Here's the drawing with two shaded views (mm, measured from the low corner). I have some questions. Give positions to 0.01 mm unless a question says otherwise; leave off trailing zeros. Write each loop counter-clockwise with the first axis right and the second up, starting at its lowest first coordinate (ties: lowest second). Pieces come first, ordered by that corner, then holes.
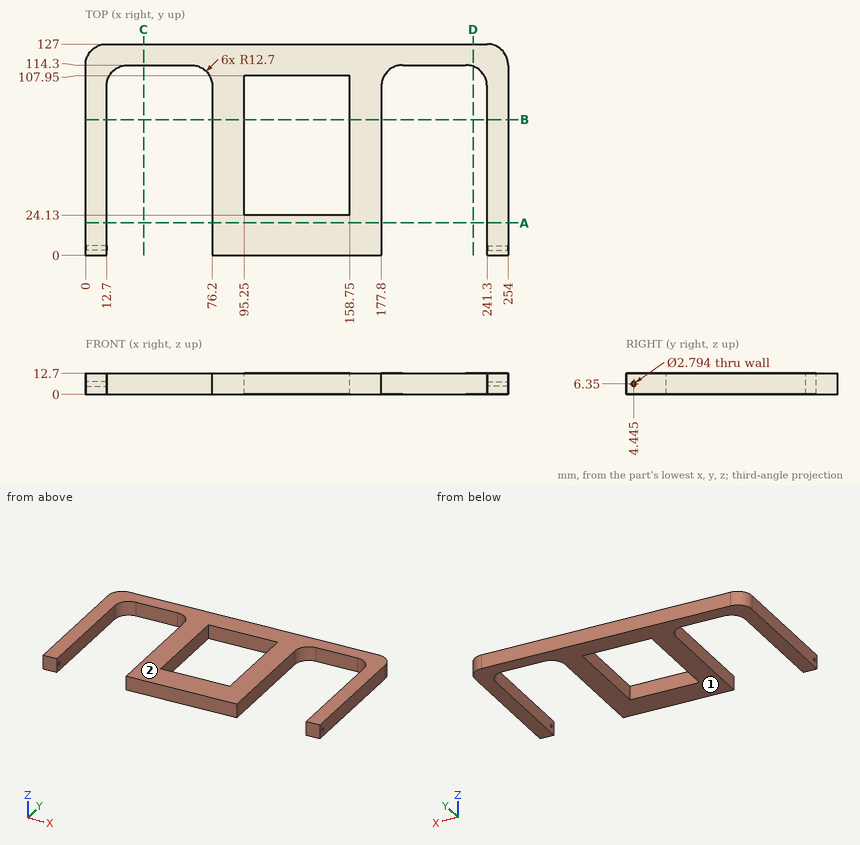
1) If we mould it in two halves opening along Z, with no side actions, what happens to the marked faces 1 and 2? For each: +Z half, -Z half, draft (parallel to the pull), parting line (faces both ways), or undercut.
Values follow:
face 1: -Z half
face 2: +Z half
2) For pin 1 Ø6.5 at (x, z) = (205.5, 4.5) entering from -Y; pin 2 Ø2.5 at (y, z) = (4.445, 6.35) entering from -X; pin 3 Ø2 at (y, z) = (4.445, 6.35) entering from +X, each with a flat end and sliding along its axis, tell me the tip position at first contact or that it passes through.
Values follow:
pin 1: stops at y = 114.3
pin 2: stops at x = 76.2
pin 3: stops at x = 177.8
3) Suppose I cut it at A-A on y = 19.5. Write out the boundary of the cut face in (x, z), plus the area to 3 significant figures.
Values follow:
outline: (0, 0) - (12.7, 0) - (12.7, 12.7) - (0, 12.7) - close; (76.2, 0) - (177.8, 0) - (177.8, 12.7) - (76.2, 12.7) - close; (241.3, 0) - (254, 0) - (254, 12.7) - (241.3, 12.7) - close
area: 1,610 mm2
4) Please list where these lines run through material, in increasing order: L1, parallel to X at y = 45, z = 5.75; L2, parallel to Y at x = 119.5, z = 5; L3, parallel to X at y = 8.5, z = 5.25.
Values follow:
L1: x = 0 to 12.7, 76.2 to 95.25, 158.75 to 177.8, 241.3 to 254
L2: y = 0 to 24.13, 107.95 to 127
L3: x = 0 to 12.7, 76.2 to 177.8, 241.3 to 254
5) Suppose I cut it at C-C on x = 35. Write out the boundary of the cut face in (y, z), plus the area to 3 significant figures.
Values follow:
outline: (114.3, 0) - (127, 0) - (127, 12.7) - (114.3, 12.7) - close
area: 161 mm2
6) Suppose I cut it at B-B on y = 81.5. Write out the boundary of the cut face in (x, z).
Values follow:
outline: (0, 0) - (12.7, 0) - (12.7, 12.7) - (0, 12.7) - close; (76.2, 0) - (95.25, 0) - (95.25, 12.7) - (76.2, 12.7) - close; (158.75, 0) - (177.8, 0) - (177.8, 12.7) - (158.75, 12.7) - close; (241.3, 0) - (254, 0) - (254, 12.7) - (241.3, 12.7) - close
7) Suppose I cut it at D-D on x = 233. Write out the boundary of the cut face in (y, z).
Values follow:
outline: (113.51, 0) - (127, 0) - (127, 12.7) - (113.51, 12.7) - close
